Part model, mm, in its own coordinate system. Coordinates: 2 decimals unless noted, no trailing zeros. Order: outer loops, then holes, each group sorted by start corner. A loop starts at its lowest first (then second) coordinate and runs counter-clockwise, first axis right, second up. Notation, with made-up numbers: (-23, 84.5) - (33, 84.5) arc R17 cw to (33, 109.5) - close; hole circle Ø11 at (-35, 57.5). An arc over 180 degrees is marked (long way). Use a Markdown table: item, result. Add a question column.
1) Saw through at C-C on y = -18. List the corners of the cut face in (x, z) (1 decimal).
2) Saw through at B-B on x = -35.5. List the corners of the cut face in (y, z).
3) Saw through at D-D on z = -0.15. Count the separate pieces of the cut face and the enclosed holes in it, then the cut area to 3 significant figures.
4) Wall check: L1, parallel to Y at x = -1.5, z = 0.95 (3 decimals); L2, parallel to X at y = -23.5, z = -1.1 (1 decimal); L3, parallel to Y at x = 9.5, z = 0.95 (3 decimals). Give the ranges that are in metal, low to high. Write a range as [from, to].
5) Drop a flat-ended pin along its axis: P1, Ø1.6, axis at y = 31.5, z = 0, coming from the +X side. Give the stop position or say it passes through.
6) Saw through at A-A on y = 22. List the corners of the cut face in (x, z) (1 decimal).
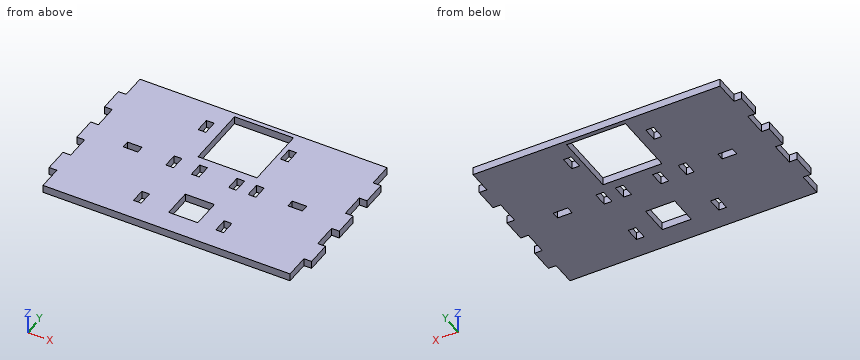
```python
from build123d import *

# Parameters (mm, degrees)
SKETCH1_W           = 6
SKETCH1_H           = 3.125
SKETCH1_W_2         = 3.175
SKETCH1_H_2         = 6
BOSS_EXTRUDE1_DEPTH = 1.5875


with BuildPart() as part:
    # Sketch1 → Boss-Extrude1 (new body, symmetric)
    with BuildSketch(Plane.XY):
        Polygon((54.175, 0), (54.175, 5), (51, 5), (51, 15), (54.175, 15), (54.175, 25), (51, 25), (51, 35), (17, 35), (0, 35), (-17, 35), (-51, 35), (-51, 25), (-54.175, 25), (-54.175, 15), (-51, 15), (-51, 5), (-54.175, 5), (-54.175, -5), (-51, -5), (-51, -15), (-54.175, -15), (-54.175, -25), (-51, -25), (-51, -35), (0, -35), (51, -35), (51, -25), (54.175, -25), (54.175, -15), (51, -15), (51, -5), (54.175, -5), align=None)
        Polygon((-18.5875, -23.333333333), (-18.5875, -20.333333333), (-15.4125, -20.333333333), (-15.4125, -26.333333333), (-18.5875, -26.333333333), align=None, mode=Mode.SUBTRACT)
        Polygon((-4.247592219, -14), (3.252407781, -14), (7.752407781, -14), (7.752407781, -26), (3.252407781, -26), (-4.247592219, -26), align=None, mode=Mode.SUBTRACT)
        Polygon((18.5875, -20.333333333), (18.5875, -23.333333333), (18.5875, -26.333333333), (15.4125, -26.333333333), (15.4125, -20.333333333), align=None, mode=Mode.SUBTRACT)
        with Locations((-34, 0)):
            Rectangle(SKETCH1_W, SKETCH1_H, mode=Mode.SUBTRACT)
        with Locations((-17, 0)):
            Rectangle(SKETCH1_W_2, SKETCH1_H_2, mode=Mode.SUBTRACT)
        with Locations((-6.422592219, 0)):
            Rectangle(SKETCH1_W_2, SKETCH1_H_2, mode=Mode.SUBTRACT)
        Polygon((-18.5875, 20.333333333), (-18.5875, 23.333333333), (-18.5875, 26.333333333), (-15.4125, 26.333333333), (-15.4125, 20.333333333), align=None, mode=Mode.SUBTRACT)
        with Locations((8.927407781, 0)):
            Rectangle(SKETCH1_W_2, SKETCH1_H_2, mode=Mode.SUBTRACT)
        with Locations((17, 0)):
            Rectangle(SKETCH1_W_2, SKETCH1_H_2, mode=Mode.SUBTRACT)
        Polygon((37, 1.5625), (37, 0), (37, -1.5625), (31, -1.5625), (31, 1.5625), align=None, mode=Mode.SUBTRACT)
        Polygon((-10.922592219, 33.175), (3.252407781, 33.175), (13.427407781, 33.175), (13.427407781, 6.825), (1.252407781, 6.825), (-10.922592219, 6.825), align=None, mode=Mode.SUBTRACT)
        Polygon((18.5875, 23.333333333), (18.5875, 20.333333333), (15.4125, 20.333333333), (15.4125, 26.333333333), (18.5875, 26.333333333), align=None, mode=Mode.SUBTRACT)
    extrude(amount=BOSS_EXTRUDE1_DEPTH, both=True)


solid = part.part
```
Results are:
| question | item | result |
|---|---|---|
| 1 | outline | (-54.2, -1.6) - (-4.2, -1.6) - (-4.2, 1.6) - (-54.2, 1.6) - close; (7.8, -1.6) - (54.2, -1.6) - (54.2, 1.6) - (7.8, 1.6) - close |
| 2 | outline | (-35, -1.59) - (-1.56, -1.59) - (-1.56, 1.59) - (-35, 1.59) - close; (1.56, -1.59) - (35, -1.59) - (35, 1.59) - (1.56, 1.59) - close |
| 3 | separate pieces | 1 |
| 3 | enclosed holes | 12 |
| 3 | area | 6,350 mm2 |
| 4 | L1 | [-35, -26], [-14, 6.825], [33.175, 35] |
| 4 | L2 | [-54.2, -18.6], [-15.4, -4.2], [7.8, 15.4], [18.6, 54.2] |
| 4 | L3 | [-35, -3], [3, 6.825], [33.175, 35] |
| 5 | P1 | x = 51 |
| 6 | outline | (-54.2, -1.6) - (-18.6, -1.6) - (-18.6, 1.6) - (-54.2, 1.6) - close; (-15.4, -1.6) - (-10.9, -1.6) - (-10.9, 1.6) - (-15.4, 1.6) - close; (13.4, -1.6) - (15.4, -1.6) - (15.4, 1.6) - (13.4, 1.6) - close; (18.6, -1.6) - (54.2, -1.6) - (54.2, 1.6) - (18.6, 1.6) - close |
